Verification items for this drawing (mm, ordinates from the low corner). A direction names the side the tool comes from. Coordinates: 2 decimals unless noted, no trailing zeros. Write each loop counter-clockwise with the first axis right and the second up, starting at its lowest first coordinate (ties: lowest second). Pieces come first, ordered by that corner, then holes. Notation, with made-up numbers: M 75.25,-38.75 L 80.25,-38.75 A20 ccw 80.25,0.25 Z; hole C 24.25,70.5 d6. An arc over 180 degrees is marked long. Put each result on its own line as item: value. Start each with the question number.
1) Mould release check, pull along X, two halves, no side actions. Record for the marked faces 4, 5 and 6: released by +X, released by -X, zero draft, split by the parting line, or undercut.
2) Scan lines: line 1 along Y through (x, z) = (5, 2.1); line 2 along X through (y, z) = (25, 10.5); line 3 along Y through (x, z) = (25, 4.4). Record each from-to range of solid material in increasing order.
3) Set-up check for the marked faces 1, 2 and 3: record each of +Z, -Z, +X, -X, +Y, -Y from which the full face is reachable in a straight line by a thin tool's end or side.
4) Gauge pin test, flat ends, axial feed: pin 1 (9.5 mm diameter, centred on x = 25, y = 25, fed in from +Z); pin 2 (3 mm diameter, centred on x = 45, y = 3.75, fed in from +Z); pin 3 (3 mm diameter, centred on y = 32.5, z = 9.5, fed in from +X); pin 4 (10 mm diameter, centred on x = 36, y = 5, fed in from +Z). Record the tip position at first contact, or that the pin passes through.
5) Cross-section at D-D on y = 30.5. Record the cut outline in (x, z), plus the area to 3 significant figures.
6) Cross-section at C-C on x = 25. Record the cut outline in (y, z).
7) Cross-section at B-B on z = 1.25. Record the cut outline in (x, y), plus the area to 3 significant figures.
8) Cross-section at A-A on x = 5. Record the cut outline in (y, z).
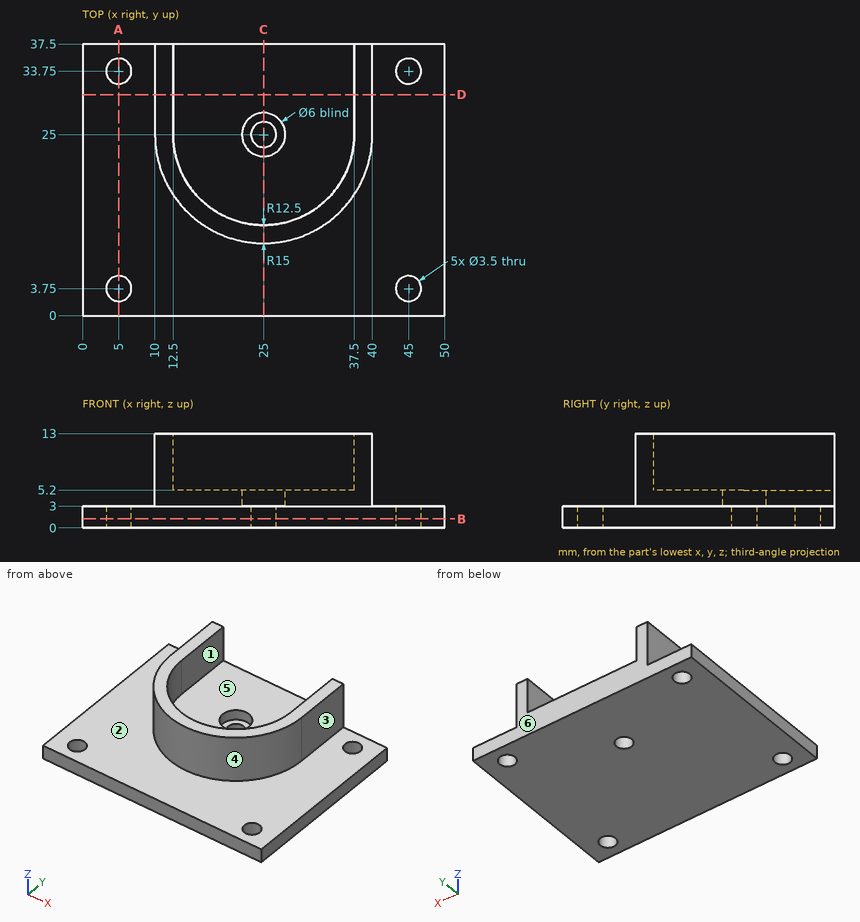
Answer key:
1. face 4: split by the parting line
1. face 5: undercut
1. face 6: zero draft
2. line 1: y = 0 to 2, 5.5 to 32, 35.5 to 37.5
2. line 2: x = 10 to 12.5, 37.5 to 40
2. line 3: y = 10 to 22, 28 to 37.5
3. face 1: +Z, +Y
3. face 2: +Z, -Y
3. face 3: +Z, +X, +Y, -Y
4. pin 1: stops at z = 5.2
4. pin 2: passes through
4. pin 3: stops at x = 40
4. pin 4: stops at z = 3
5. outline: M 0,0 L 50,0 L 50,3 L 40,3 L 40,13 L 37.5,13 L 37.5,5.2 L 12.5,5.2 L 12.5,13 L 10,13 L 10,3 L 0,3 Z
5. area: 255 mm²
6. outline: M 0,0 L 23.25,0 L 23.25,3 L 22,3 L 22,5.2 L 12.5,5.2 L 12.5,13 L 10,13 L 10,3 L 0,3 Z; M 26.75,0 L 37.5,0 L 37.5,5.2 L 28,5.2 L 28,3 L 26.75,3 Z
7. outline: M 0,0 L 50,0 L 50,37.5 L 0,37.5 Z; hole C 5,3.75 d3.5; hole C 5,33.75 d3.5; hole C 25,25 d3.5; hole C 45,3.75 d3.5; hole C 45,33.75 d3.5
7. area: 1,830 mm²
8. outline: M 0,0 L 2,0 L 2,3 L 0,3 Z; M 5.5,0 L 32,0 L 32,3 L 5.5,3 Z; M 35.5,0 L 37.5,0 L 37.5,3 L 35.5,3 Z
